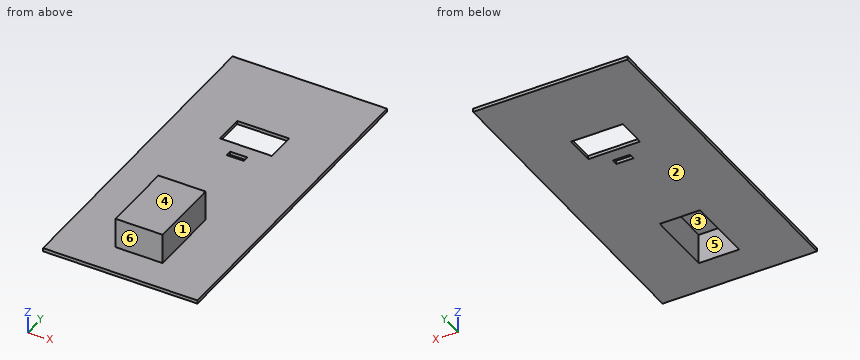
from build123d import *

# Parameters (mm, degrees)
SKETCH1_W           = 575
SKETCH1_H           = 1219.2
BOSS_EXTRUDE1_DEPTH = 12.7
SKETCH2_W           = 193
SKETCH2_H           = 111
SKETCH2_W_2         = 64
SKETCH2_H_2         = 22.19
CUT_EXTRUDE1_DEPTH  = 12.7
SKETCH3_W           = 150
SKETCH3_H           = 250
CUT_EXTRUDE2_DEPTH  = 12.7
SKETCH4_W           = 175.4
SKETCH4_H           = 275.4
SKETCH4_W_2         = 150
SKETCH4_H_2         = 250
BOSS_EXTRUDE2_DEPTH = 100
SKETCH5_W           = 175.4
SKETCH5_H           = 275.4
BOSS_EXTRUDE3_DEPTH = 12.7


with BuildPart() as part:
    # Sketch1 → Boss-Extrude1 (new body)
    with BuildSketch(Plane.XY):
        Rectangle(SKETCH1_W, SKETCH1_H)
    extrude(amount=BOSS_EXTRUDE1_DEPTH)

    # Sketch2 → Cut-Extrude1 (cut)
    with BuildSketch(Plane.XY.offset(12.7)):
        with Locations((0, 254.1)):
            Rectangle(SKETCH2_W, SKETCH2_H)
        with Locations((0, 141.033454098)):
            Rectangle(SKETCH2_W_2, SKETCH2_H_2)
    extrude(amount=-CUT_EXTRUDE1_DEPTH, mode=Mode.SUBTRACT)

    # Sketch3 → Cut-Extrude2 (cut)
    with BuildSketch(Plane(origin=(0, 0, 0), x_dir=(-1, 0, 0), z_dir=(0, 0, -1))):
        with Locations((0, -350.163151911)):
            Rectangle(SKETCH3_W, SKETCH3_H)
    extrude(amount=-CUT_EXTRUDE2_DEPTH, mode=Mode.SUBTRACT)

    # Sketch4 → Boss-Extrude2 (add)
    with BuildSketch(Plane.XY.offset(12.7)):
        with Locations((0, -350.163151911)):
            Rectangle(SKETCH4_W, SKETCH4_H)
        with Locations((0, -350.163151911)):
            Rectangle(SKETCH4_W_2, SKETCH4_H_2, mode=Mode.SUBTRACT)
    extrude(amount=BOSS_EXTRUDE2_DEPTH)

    # Sketch5 → Boss-Extrude3 (add)
    with BuildSketch(Plane.XY.offset(112.7)):
        with Locations((0, -350.163151911)):
            Rectangle(SKETCH5_W, SKETCH5_H)
    extrude(amount=BOSS_EXTRUDE3_DEPTH)


solid = part.part
Geometry: final body of the model. Coordinates: model frame, mm. Face numbers are marked on the shaded views. A direction names the side the tool comes from. Coordinates: 2 decimals unless noted, no trailing zeros. Order: outer loops, then holes, each group sorted by start corner. A loop starts at its lowest first (then second) coordinate and runs counter-clockwise, first axis right, second up.
1) Section A-A (x = 9). Return loops of the section in (y, z).
Result sheet:
outline: (-609.6, 0) - (-475.16, 0) - (-475.16, 112.7) - (-225.16, 112.7) - (-225.16, 0) - (129.94, 0) - (129.94, 12.7) - (-212.46, 12.7) - (-212.46, 125.4) - (-487.86, 125.4) - (-487.86, 12.7) - (-609.6, 12.7) - close; (152.13, 0) - (198.6, 0) - (198.6, 12.7) - (152.13, 12.7) - close; (309.6, 0) - (609.6, 0) - (609.6, 12.7) - (309.6, 12.7) - close
2) Ray query, probe 1 along X at (y, z) = (-366, 28); probe 2 along Y at (x, z) = (-60, 82); probe 3 along Z at (x, y) = (-74.5, -515). Return the intervals inside material, ascending.
Result sheet:
probe 1: x = -87.7 to -75, 75 to 87.7
probe 2: y = -487.86 to -475.16, -225.16 to -212.46
probe 3: z = 0 to 12.7
3) Section B-B (z = 70.5). Return loops of the section in (x, y), then the cut area to 3 significant figures.
Result sheet:
outline: (-87.7, -487.86) - (87.7, -487.86) - (87.7, -212.46) - (-87.7, -212.46) - close; hole (-75, -475.16) - (75, -475.16) - (75, -225.16) - (-75, -225.16) - close
area: 10,800 mm2
4) Section C-C (y = -339). Return loops of the section in (x, z).
Result sheet:
outline: (-287.5, 0) - (-75, 0) - (-75, 112.7) - (75, 112.7) - (75, 0) - (287.5, 0) - (287.5, 12.7) - (87.7, 12.7) - (87.7, 125.4) - (-87.7, 125.4) - (-87.7, 12.7) - (-287.5, 12.7) - close
5) Section D-D (x = -180.5). Return loops of the section in (y, z).
Result sheet:
outline: (-609.6, 0) - (609.6, 0) - (609.6, 12.7) - (-609.6, 12.7) - close
6) Set-up query: the marked faces 1, 2 and 3. Return all of +Z, -Z, +X, -X, +Y, -Y with unobstructed straight access to the full face (end or side cutting, diameter ignored); none if empty.
Result sheet:
face 1: +Z, +X, +Y, -Y
face 2: -Z, +X, -X, +Y, -Y
face 3: -Z
7) Draft query along Y for the marked faces 4, 5 and 6. Return one class per face: released by +Y, released by -Y, zero draft, split by the parting line, or undercut.
Result sheet:
face 4: zero draft
face 5: undercut
face 6: released by -Y
8) First-contact query: P1, Ø8, axis at y = -213, z = 49.5, coming from the -X side; P2, Ø1, axis at x = -161, y = -259, coming from the -Z side; P3, Ø6, axis at y = -414, z = 70.5, coming from the +X side; P4, Ø5, axis at x = -48, z = 69.5, coming from the +Y side. Flat tips, straight axial feed; report the tip coordinate or a pass-through.
Result sheet:
P1: stops at x = -87.7
P2: stops at z = 0
P3: stops at x = 87.7
P4: stops at y = -212.46
